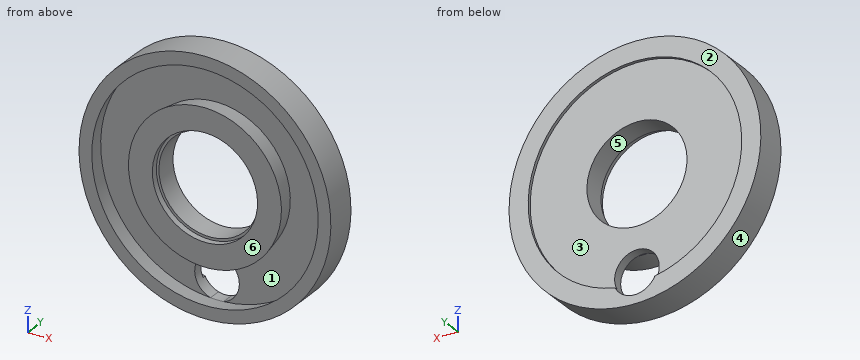
```python
from build123d import *

# Parameters (mm, degrees)
F2_R     = 7
F3_DEPTH = 4.001


# Not quite as in the source:
# - a feature names something its author has since deleted; it is built from what else it names


with BuildPart() as f1:
    # F0 (on Right) → F1 (revolve)
    with BuildSketch(Plane.YZ):
        Polygon((-59.0552871114, 24), (-59.0552871114, 16.5), (-57.0552871114, 16.5), (-57.0552871114, 15.7), (-50.0552871114, 15.7), (-50.0552871114, 33.5), (-49.0552871114, 33.5), (-49.0552871114, 39.5), (-59.0552871114, 39.5), (-59.0552871114, 35.5), (-53.0552871114, 36.5), (-53.0552871114, 23), align=None)
    revolve(axis=Axis((0, -43.8180491328, 0), (0, 1, 0)))

    # F2 (on face) → F3 (cut, through all)
    with BuildSketch(Plane.XZ.offset(53.0552871114)):
        with Locations((0, -29.75)):
            Circle(F2_R)
        with BuildLine():
            ThreePointArc((-2.0528271341, -36.4422268908), (0, -36.75), (2.0528271341, -36.4422268908))
            ThreePointArc((2.0528271341, -36.4422268908), (0, -36.5), (-2.0528271341, -36.4422268908))
        make_face()
    extrude(amount=-F3_DEPTH, mode=Mode.SUBTRACT)


solid = f1.part
```
Here's how the part is built. I have some questions about the finished solid (model axes, mm). Face numbers are marked on the shaded views. A direction names the side the tool comes from. Round coordinates to 2 decimals unless told otherwise and drop trailing zeros. Order: outer loops, then holes, each group sorted by start corner. A loop starts at its lowest first (then second) coordinate and runs counter-clockwise, first axis right, second up. Notation, with made-up numbers: (56, 19) -> (92, 19) arc R25 ccw to (92, 44) -> close; hole circle Ø7 at (13.25, -21.75). An arc over 180 degrees is marked (long way). Use a Markdown table: item, result. Add a question column.
(1) Suppose I cut it at B-B, the plane x = 0. Please give me the cut outline in (y, z).
(2) For the marked faces 1, 2 and 3, which set-ups out of +Z, -Z, +X, -X, +Y, -Y let a thin tool reach every point of the face, with its end or its side?
(3) Suppose I cut it at C-C, the plane y = -55.5. Please give me the cut outline in (x, z).
(4) Suppose I cut it at A-A, the plane z = 0. Please give me the cut outline in (x, y).
(5) If we mould it in two halves opening along X, with no side actions, what happens to the marked faces 4, 5 and 6? For each: released by +X, released by -X, zero draft, split by the parting line, or undercut.
(6) I need wall thicknesses on line 1 along Z through (x, y) = (14, -55); line 2 along X through (y, z) = (-49.25, 0); line 3 along Z through (x, y) = (19.5, -57.5). Which ranges of each line are inside material? Lowest first, please.
(7) For pin 1 Ø4 at (x, y) = (-7.5, -57.5) entering from +Z; pin 2 Ø6 at (y, z) = (-56, -27) entering from -X; pin 3 Ø6 at (x, y) = (13.5, -54.5) entering from +Z, each with a flat end and sliding along its axis, tell me the tip position at first contact or that it passes through.
Verdict:
| question | item | result |
|---|---|---|
| 1 | outline | (-59.06, -39.5) -> (-49.06, -39.5) -> (-49.06, -36.75) -> (-53.06, -36.75) -> (-53.06, -36.5) -> (-59.06, -35.5) -> close; (-59.06, -24) -> (-53.06, -23) -> (-53.06, -22.75) -> (-50.06, -22.75) -> (-50.06, -15.7) -> (-57.06, -15.7) -> (-57.06, -16.5) -> (-59.06, -16.5) -> close; (-59.06, 16.5) -> (-57.06, 16.5) -> (-57.06, 15.7) -> (-50.06, 15.7) -> (-50.06, 33.5) -> (-49.06, 33.5) -> (-49.06, 39.5) -> (-59.06, 39.5) -> (-59.06, 35.5) -> (-53.06, 36.5) -> (-53.06, 23) -> (-59.06, 24) -> close |
| 2 | face 1 | none |
| 2 | face 2 | +Z, -Z, +X, -X, +Y |
| 2 | face 3 | +Y |
| 3 | outline | circle Ø79 at (0, 0); circle Ø46.81 at (0, 0); hole circle Ø72.19 at (0, 0); hole circle Ø31.4 at (0, 0) |
| 4 | outline | (-39.5, -59.06) -> (-35.5, -59.06) -> (-36.5, -53.06) -> (-23, -53.06) -> (-24, -59.06) -> (-16.5, -59.06) -> (-16.5, -57.06) -> (-15.7, -57.06) -> (-15.7, -50.06) -> (-33.5, -50.06) -> (-33.5, -49.06) -> (-39.5, -49.06) -> close; (15.7, -57.06) -> (16.5, -57.06) -> (16.5, -59.06) -> (24, -59.06) -> (23, -53.06) -> (36.5, -53.06) -> (35.5, -59.06) -> (39.5, -59.06) -> (39.5, -49.06) -> (33.5, -49.06) -> (33.5, -50.06) -> (15.7, -50.06) -> close |
| 5 | face 4 | split by the parting line |
| 5 | face 5 | undercut |
| 5 | face 6 | zero draft |
| 6 | line 1 | -36.94 to -33.36, -18.66 to -7.11, 7.11 to 18.66, 33.36 to 36.94 |
| 6 | line 2 | -39.5 to -33.5, 33.5 to 39.5 |
| 6 | line 3 | -34.35 to -29.97, -13.54 to 13.54, 29.97 to 34.35 |
| 7 | pin 1 | z = 39.12 |
| 7 | pin 2 | x = -31.37 |
| 7 | pin 3 | z = 38.08 |
